Source: CAD feature listing. Evaluate the final solid. Frame: model axes, mm. A direction names the side the tool comes from. Give positions to 0.01 mm unless a question says otherwise; leave off trailing zeros. Order: outer loops, then holes, each group sorted by start corner. A loop starts at its lowest first (then second) coordinate and runs counter-clockwise, first axis right, second up. Notation, with made-up numbers: M -23.5,-17.5 L -0.5,-17.5 A17 ccw -0.5,14.5 Z; hole C -22.5,33 d2. An arc over 180 degrees is marked long. Answer as a JSON object with one key per item and string values. Group by question number.
1. Set-up query: faces 5 (the cylindrical face through (-1.915, 30.412, 6.152)), 6 (the flat face through (0, 0, 0)). Return all of +Z, -Z, +X, -X, +Y, -Y with unobstructed straight access to the full face (end or side cutting, diameter ignored); none if empty.
2. Pin query (flat end, axial travel): P1, Ø4, axis at x = 13.5, z = 5, coming from the +Y side; P2, Ø3, axis at x = 0, z = 7.62, coming from the +Y side; P3, Ø6, axis at x = 37.38, y = -11.32, coming from the +Z side; P4, Ø8, axis at x = 5.5, z = 8.5, coming from the -Y side. Return the tip coordinate at first contact, or that it passes through.
3. Section query A-A (y = 0). Output: boundary loops of the cut face in (x, z).
4. Pull-direction query (Z, two-part tool) for faces 1 (the cylindrical face through (35.33, -12.17, -2.58)), 2 (the cylindrical face through (-1.915, -30.449, 6.152)), 3 (the flat face through (-1, 1, -5.08)), 4 (the cylindrical face through (-30.413, -1.915, 6.152)); classes: +Z half, -Z half, draft (parallel to the pull), parting line (faces both ways), or undercut.
5. Material intervals for L1, parallel to Z at x = -26.5, y = -31; L2, parallel to Z at x = 0, y = 30; L3, parallel to X at y = 6, z = 13, sorted ascending. Write a range as [from, to].
6. Section query C-C (z = 7.62). Output: boundary loops of the cut face in (x, y), plus the area to 3 significant figures.
7. Section query D-D (z = 2.25). Output: boundary loops of the cut face in (x, y).
from build123d import *

# Parameters (mm, degrees)
F0_R      = 31.75
F0_R_2    = 29.21
F1_DEPTH  = 13.97
F4_R      = 44.9
F5_DEPTH  = 5.08
F6_R      = 2.413
F7_DEPTH  = 38.1
F9_D      = 4.445
F9_DEPTH  = 12.7
F10_R     = 2.413
F11_DEPTH = 50.8


with BuildPart() as f1:
    # F0 (on Top) → F1 (new body)
    with BuildSketch(Plane.XY):
        Circle(F0_R)
        Circle(F0_R_2, mode=Mode.SUBTRACT)
    extrude(amount=F1_DEPTH)

    # F4 (on Top) → F5 (join)
    with BuildSketch(Plane.XY):
        Circle(F4_R)
    extrude(amount=-F5_DEPTH)

    # F6 (on Front) → F7 (cut, symmetric)
    with BuildSketch(Plane.XZ):
        with Locations((0, 7.62)):
            Circle(F6_R)
    extrude(amount=F7_DEPTH, both=True, mode=Mode.SUBTRACT)

    # F9
    with Locations(Plane.XY):
        with Locations((-8.89, 38.032818), (-28.492387, -26.715375), (37.382387, -11.317443)):
            Hole(F9_D / 2, depth=F9_DEPTH)

    # F10 (on Right) → F11 (cut, symmetric)
    with BuildSketch(Plane.YZ):
        with Locations((0, 7.62)):
            Circle(F10_R)
    extrude(amount=F11_DEPTH, both=True, mode=Mode.SUBTRACT)


solid = f1.part
Answer sheet:
{
 "1": {"face 5": "+Y, -Y", "face 6": "+Z"},
 "2": {"P1": "y = 29.59", "P2": "through", "P3": "z = 0", "P4": "y = -31.71"},
 "3": {"outline": "M -44.9,-5.08 L 44.9,-5.08 L 44.9,0 L 31.75,0 L 31.75,5.21 L 29.21,5.21 L 29.21,0 L -29.21,0 L -29.21,5.21 L -31.75,5.21 L -31.75,0 L -44.9,0 Z; M -31.75,10.03 L -29.21,10.03 L -29.21,13.97 L -31.75,13.97 Z; M 29.21,10.03 L 31.75,10.03 L 31.75,13.97 L 29.21,13.97 Z"},
 "4": {"face 1": "draft", "face 2": "undercut", "face 3": "-Z half", "face 4": "undercut"},
 "5": {"L1": "[-5.08, 0]", "L2": "[-5.08, 5.21], [10.03, 13.97]", "L3": "[-31.18, -28.59], [28.59, 31.18]"},
 "6": {"outline": "M -31.66,-2.41 A31.75 ccw -2.41,-31.66 L -2.41,-29.11 A29.21 cw -29.11,-2.41 Z; M -31.66,2.41 L -29.11,2.41 A29.21 cw -2.41,29.11 L -2.41,31.66 A31.75 ccw Z; M 2.41,-31.66 A31.75 ccw 31.66,-2.41 L 29.11,-2.41 A29.21 cw 2.41,-29.11 Z; M 2.41,29.11 A29.21 cw 29.11,2.41 L 31.66,2.41 A31.75 ccw 2.41,31.66 Z", "area": "437 mm^2"},
 "7": {"outline": "C 0,0 d63.5; hole C 0,0 d58.42"}
}
